from build123d import *

# Parameters (mm, degrees)
SKETCH_1_W          = 92
SKETCH_1_H          = 50
SKETCH_1_R          = 1.55
SKETCH_1_R_2        = 10.5
SKETCH_1_R_3        = 2.05
EXTRUDE_1_DEPTH     = 4
SKETCH_13_W         = 8
SKETCH_13_H         = 50
CUT_EXTRUDE_8_DEPTH = 4
FILLET2_R           = 4
SKETCH1_R           = 6
CUT_EXTRUDE1_DEPTH  = 5


with BuildPart() as part:
    # 草图1 → 凸台-拉伸1 (new, symmetric)
    with BuildSketch(Plane(origin=(0, 0, 0), x_dir=(1, 0, 0), z_dir=(0, 1, 0))):
        Rectangle(SKETCH_1_W, SKETCH_1_H)
        with Locations(Location((-42, -21, 0), (0, 0, 270))):
            Circle(SKETCH_1_R, mode=Mode.SUBTRACT)
        with Locations(Location((0, 0, 0), (0, 0, 270))):
            Circle(SKETCH_1_R_2, mode=Mode.SUBTRACT)
        with Locations(Location((0, -20, 0), (0, 0, 270))):
            Circle(SKETCH_1_R_3, mode=Mode.SUBTRACT)
        with Locations(Location((-17.320508076, 10, 0), (0, 0, 270))):
            Circle(SKETCH_1_R_3, mode=Mode.SUBTRACT)
        with Locations(Location((17.320508076, 10, 0), (0, 0, 270))):
            Circle(SKETCH_1_R_3, mode=Mode.SUBTRACT)
        with Locations(Location((42, -21, 0), (0, 0, 90))):
            Circle(SKETCH_1_R, mode=Mode.SUBTRACT)
        with Locations(Location((42, 21, 0), (0, 0, 270))):
            Circle(SKETCH_1_R, mode=Mode.SUBTRACT)
        with Locations(Location((-42, 21, 0), (0, 0, 90))):
            Circle(SKETCH_1_R, mode=Mode.SUBTRACT)
        with Locations(Location((0, 18, 0), (0, 0, 270))):
            Circle(SKETCH_1_R, mode=Mode.SUBTRACT)
        with Locations(Location((15.588457268, -9, 0), (0, 0, 270))):
            Circle(SKETCH_1_R, mode=Mode.SUBTRACT)
        with Locations(Location((-15.588457268, -9, 0), (0, 0, 270))):
            Circle(SKETCH_1_R, mode=Mode.SUBTRACT)
    extrude(amount=EXTRUDE_1_DEPTH, both=True)

    # 草图13 → 切除-拉伸8 (cut)
    with BuildSketch(Plane.XZ.offset(4)):
        with Locations((42, 0)):
            Rectangle(SKETCH_13_W, SKETCH_13_H)
        with Locations((-42, 0)):
            Rectangle(SKETCH_13_W, SKETCH_13_H)
    extrude(amount=-CUT_EXTRUDE_8_DEPTH, mode=Mode.SUBTRACT)

    # Fillet2
    fillet2_edges = [part.edges().sort_by_distance(p)[0] for p in [
        (46, 2, -25),
        (46, 2, 25),
        (-46, 2, -25),
        (-46, 2, 25),
    ]]
    fillet(fillet2_edges, radius=FILLET2_R)

    # Sketch1 → Cut-Extrude1 (cut)
    with BuildSketch(Plane(origin=(0, -4, 0), x_dir=(-1, 0, 0), z_dir=(0, -1, 0))):
        with Locations(Location((0, 18, 0), (0, 0, 90))):
            Circle(SKETCH1_R)
        with Locations(Location((15.588457268, -9, 0), (0, 0, 90))):
            Circle(SKETCH1_R)
        with Locations(Location((-15.588457268, -9, 0), (0, 0, 90))):
            Circle(SKETCH1_R)
    extrude(amount=-CUT_EXTRUDE1_DEPTH, mode=Mode.SUBTRACT)


solid = part.part
For this review, take the finished solid that the model builds, in its own axes (mm). A direction names the side the tool comes from. Coordinates: 2 decimals unless noted, no trailing zeros. Order: outer loops, then holes, each group sorted by start corner. A loop starts at its lowest first (then second) coordinate and runs counter-clockwise, first axis right, second up. Notation, with made-up numbers: (10.5, -11.5) - (18.5, -11.5) arc R12 ccw to (18.5, 2.5) - close; hole circle Ø2 at (62.5, -15). An arc over 180 degrees is marked (long way). Answer as CSV lines item,"result". Start each with the question number.
1) Add section B-B (y = -2). State the section outline as (x, z) points.
2) Add section C-C (z = -18). State the section outline as (x, y) points.
3) Add section D-D (y = 3). Count the separate pieces of the cut face and the enclosed holes in it, then the cut area to 3 significant figures.
4) Machinability: for faces 1 (the flat face through (-1.25, 1, -19.25)), 2 (the flat face through (-42, 0, 0)), 3 (the flat face through (38, -2, 0)), 4 (the cylindrical face through (-17.23, -0.06, -12.05)), which of the approach directions +Z, -Z, +X, -X, +Y, -Y give a long, thin tool a straight path to every point of the face, cutting with its end or side? Answer none if there is none.
5) Draft analysis for pull direction Z (two halves, no side actions). For faces 5 (the flat face through (46, 2, 0)), 6 (the cylindrical face through (44.797, 2.028, 23.859)), 7 (the cylindrical face through (40.625, 1.972, -20.285)), 8 (the cylindrical face through (43.375, 1.972, 20.285)), state which applies: +Z half, -Z half, draft (parallel to the pull), parting line (faces both ways), or undercut.
6) Add section A-A (z = 0). State the section outline as (x, y) points, then the cut area to 3 significant figures.
7) To check wall thickness, follow line 1 along Z through (x, y) = (42, 1.65); line 2 along X through (y, z) = (1.75, -21); line 3 along X through (y, z) = (0.75, 9). State the ranges of each line that lie inside material, in increasing order. Write a range as [from, to].
8) Insertion check: P1, Ø4.5, axis at y = -2.5, z = -6, coming from the +X side; P2, Ø2, axis at y = -2.5, z = -4.5, coming from the -X side; P3, Ø4, axis at x = 15.59, z = 9, coming from the -Y side. Each pin has a flat end and moves straight along its axis. Give the tip position at first contact, or say it passes through.
Result:
1,outline,"(-38, -25) - (38, -25) - (38, 25) - (-38, 25) - close; hole circle Ø12 at (-15.59, 9); hole circle Ø4.1 at (-17.32, -10); hole circle Ø21 at (0, 0); hole circle Ø12 at (0, -18); hole circle Ø4.1 at (0, 20); hole circle Ø12 at (15.59, 9); hole circle Ø4.1 at (17.32, -10)"
2,outline,"(-46, 0) - (-38, 0) - (-38, -4) - (-6, -4) - (-6, 1) - (-1.55, 1) - (-1.55, 4) - (-46, 4) - close; (1.55, 1) - (6, 1) - (6, -4) - (38, -4) - (38, 0) - (46, 0) - (46, 4) - (1.55, 4) - close"
3,separate pieces,"1"
3,enclosed holes,"11"
3,area,"4,150 mm^2"
4,face 1,"-Y"
4,face 2,"+Z, -Z, -X, -Y"
4,face 3,"+Z, -Z, +X, -Y"
4,face 4,"+Y, -Y"
5,face 5,"draft"
5,face 6,"+Z half"
5,face 7,"undercut"
5,face 8,"undercut"
6,outline,"(-46, 0) - (-38, 0) - (-38, -4) - (-10.5, -4) - (-10.5, 4) - (-46, 4) - close; (10.5, -4) - (38, -4) - (38, 0) - (46, 0) - (46, 4) - (10.5, 4) - close"
6,area,"504 mm^2"
7,line 1,"[-25, -22.55], [-19.45, 19.45], [22.55, 25]"
7,line 2,"[-46, -43.55], [-40.45, 40.45], [43.55, 46]"
7,line 3,"[-46, -21.59], [-9.59, -5.41], [5.41, 9.59], [21.59, 46]"
8,P1,"x = 38"
8,P2,"x = -38"
8,P3,"y = 1"
